```python
from build123d import *

# Parameters (mm, degrees)
SKETCH1_R           = 75.5
BOSS_EXTRUDE1_DEPTH = 15.2
SKETCH2_R           = 15.2
CUT_EXTRUDE1_DEPTH  = 9
CHAMFER1_SIZE       = 1
SKETCH4_R           = 5
CUT_EXTRUDE2_DEPTH  = 28
CHAMFER2_SIZE       = 1


with BuildPart() as part:
    # Sketch1 → Boss-Extrude1 (new body)
    with BuildSketch(Plane(origin=(0, 0, 0), x_dir=(1, 0, 0), z_dir=(0, 1, 0))):
        with Locations(Location((0, 0, 0), (0, 0, 90))):
            Circle(SKETCH1_R)
    extrude(amount=BOSS_EXTRUDE1_DEPTH)

    # Sketch2 → Cut-Extrude1 (cut)
    with BuildSketch(Plane.XZ):
        with Locations(Location((0, 0, 0), (0, 0, 270))):
            Circle(SKETCH2_R)
    extrude(amount=-CUT_EXTRUDE1_DEPTH, mode=Mode.SUBTRACT)

    # Chamfer1
    chamfer1_edges = [part.edges().sort_by_distance(p)[0] for p in [
        (0, 0, 15.2),
    ]]
    chamfer(chamfer1_edges, length=CHAMFER1_SIZE)

    # Sketch4 → Cut-Extrude2 (cut)
    with BuildSketch(Plane.XZ.offset(-9)):
        with Locations(Location((0, 0, 0), (0, 0, 270))):
            Circle(SKETCH4_R)
    extrude(amount=-CUT_EXTRUDE2_DEPTH, mode=Mode.SUBTRACT)

    # Chamfer2
    chamfer2_edges = [part.edges().sort_by_distance(p)[0] for p in [
        (0, 0, 75.5),
        (0, 15.2, 75.5),
    ]]
    chamfer(chamfer2_edges, length=CHAMFER2_SIZE)


solid = part.part
```
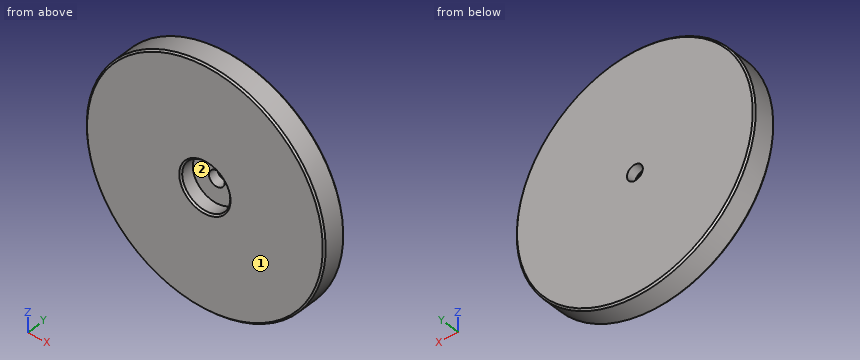
Verification items for the finished model (mm, model axes). Face numbers are marked on the shaded views. A direction names the side the tool comes from. Coordinates: 2 decimals unless noted, no trailing zeros. Loops run counter-clockwise (first coordinate to the right, second up) from the corner with the lowest first, then second, coordinate; pieces in that order, holes last. Notation, with made-up numbers: (13, 26) - (68, 26) arc R20 cw to (68, 47) - close; hole circle Ø10 at (45, -27.75). An arc over 180 degrees is marked (long way). Return JSON: item names as keys, results as strings.
1. Section check B-B, the plane z = 0. Record the boundary of the cut face in (x, y).
Established:
{"outline": "(-75.5, 1) - (-74.5, 0) - (-16.2, 0) - (-15.2, 1) - (-15.2, 9) - (-5, 9) - (-5, 15.2) - (-74.5, 15.2) - (-75.5, 14.2) - close; (5, 9) - (15.2, 9) - (15.2, 1) - (16.2, 0) - (74.5, 0) - (75.5, 1) - (75.5, 14.2) - (74.5, 15.2) - (5, 15.2) - close"}
2. Thickness scan on L1, parallel to X at y = 6.75, z = 0; L2, parallel to X at y = 10.5, z = 0; L3, parallel to Z at x = -25, y = 6. Record the ranges inside material, lowest first.
Established:
{"L1": "x = -75.5 to -15.2, 15.2 to 75.5", "L2": "x = -75.5 to -5, 5 to 75.5", "L3": "z = -71.24 to 71.24"}
3. Section check A-A, the plane x = 0. Record the boundary of the cut face in (y, z).
Established:
{"outline": "(0, -74.5) - (1, -75.5) - (14.2, -75.5) - (15.2, -74.5) - (15.2, -5) - (9, -5) - (9, -15.2) - (1, -15.2) - (0, -16.2) - close; (0, 16.2) - (1, 15.2) - (9, 15.2) - (9, 5) - (15.2, 5) - (15.2, 74.5) - (14.2, 75.5) - (1, 75.5) - (0, 74.5) - close"}
4. Section check C-C, the plane y = 6.75. Record the boundary of the cut face in (x, z).
Established:
{"outline": "circle Ø151 at (0, 0); hole circle Ø30.4 at (0, 0)"}
5. Tool access check on the marked faces 1 and 2. Record the directions out of +Z, -Z, +X, -X, +Y, -Y that give a thin tool (end or side, any length) a straight path to the whole face; none if there is none.
Established:
{"face 1": "+Z, -Z, +X, -X, -Y", "face 2": "-Y"}
6. Go/stop test with flat-tipped pins: pin 1 (3 mm diameter, centred on x = -32.5, y = 10, fed in from +Z); pin 2 (5 mm diameter, centred on y = 9.5, z = 7.5, fed in from +X); pin 3 (8 mm diameter, centred on y = 12.5, z = 27, fed in from +X). Record where each tip stops, or that it passes through.
Established:
{"pin 1": "stops at z = 68.84", "pin 2": "stops at x = 75.33", "pin 3": "stops at x = 71.91"}
